Build history of the part. All positions in model axes, mm. A direction names the side the tool comes from. Coordinates: 2 decimals unless noted, no trailing zeros. Order: outer loops, then holes, each group sorted by start corner. A loop starts at its lowest first (then second) coordinate and runs counter-clockwise, first axis right, second up. Notation, with made-up numbers: (72, 53.25) - (78, 53.25) arc R12 ccw to (78, 67.25) - close; hole circle Ø1 at (19, -2.5). An arc over 180 degrees is marked (long way). Write each question's results on one line, items separated by ' | '.
from build123d import *

# Parameters (mm, degrees)
SKETCH_1_W           = 235
SKETCH_1_H           = 35
SKETCH_1_R           = 1.6
EXTRUDE_1_DEPTH      = 18
FILLET_1_R           = 1.5
CUT_EXTRUDE_1_DEPTH  = 237.337153237
SKETCH_3_W           = 13
SKETCH_3_H           = 19
CUT_EXTRUDE_2_DEPTH  = 237.337153237
SKETCH_5_R           = 1.6
CUT_EXTRUDE_5_DEPTH  = 121.151987083
SKETCH_6_R           = 3
CUT_EXTRUDE_6_DEPTH  = 10
SKETCH_10_W          = 29
SKETCH_10_H          = 35
CUT_EXTRUDE_9_DEPTH  = 30
FILLET_2_R           = 3
FILLET_5_R           = 1.5
SKETCH_11_W          = 30
SKETCH_11_H          = 19
CUT_EXTRUDE_10_DEPTH = 30
FILLET_6_R           = 5
EXTRUDE_2_DEPTH      = 10
SKETCH_13_W          = 250
SKETCH_13_H          = 88
CUT_EXTRUDE_11_DEPTH = 168.142155066


with BuildPart() as part:
    # 草图1 → 凸台-拉伸1 (new body)
    with BuildSketch(Plane.XY):
        Rectangle(SKETCH_1_W, SKETCH_1_H)
        with Locations((-47.5, 13.5)):
            Circle(SKETCH_1_R, mode=Mode.SUBTRACT)
        with Locations(Location((47.5, 13.5, 0), (0, 0, 180))):
            Circle(SKETCH_1_R, mode=Mode.SUBTRACT)
        with Locations((-47.5, 6)):
            Circle(SKETCH_1_R, mode=Mode.SUBTRACT)
        with Locations(Location((47.5, 6, 0), (0, 0, 180))):
            Circle(SKETCH_1_R, mode=Mode.SUBTRACT)
    extrude(amount=EXTRUDE_1_DEPTH)

    # 圆角1
    fillet_1_edges = [part.edges().sort_by_distance(p)[0] for p in [
        (-117.5, 17.5, 9),
        (117.5, 17.5, 9),
    ]]
    fillet(fillet_1_edges, radius=FILLET_1_R)

    # 草图2 → 切除-拉伸1 (cut, through all)
    with BuildSketch(Plane.ZY.offset(117.5)):
        Polygon((0, 1.5), (8, 17.5), (0, 17.5), align=None)
    extrude(amount=-CUT_EXTRUDE_1_DEPTH, mode=Mode.SUBTRACT)

    # 草图3 → 切除-拉伸2 (cut, through all)
    with BuildSketch(Plane.ZY.offset(117.5)):
        with Locations((11.5, -8)):
            Rectangle(SKETCH_3_W, SKETCH_3_H)
    extrude(amount=-CUT_EXTRUDE_2_DEPTH, mode=Mode.SUBTRACT)

    # 草图5 → 切除-拉伸5 (cut, through all)
    with BuildSketch(Plane(origin=(0, 0, 0), x_dir=(-1, 0, 0), z_dir=(0, 0, -1))):
        with Locations((47.5, -4.5)):
            Circle(SKETCH_5_R)
        with Locations((47.5, -12)):
            Circle(SKETCH_5_R)
        with Locations(Location((-47.5, -12, 0), (0, 0, 90))):
            Circle(SKETCH_5_R)
        with Locations(Location((-47.5, -4.5, 0), (0, 0, 90))):
            Circle(SKETCH_5_R)
    extrude(amount=-CUT_EXTRUDE_5_DEPTH, mode=Mode.SUBTRACT)

    # 草图6 → 切除-拉伸6 (cut)
    with BuildSketch(Plane(origin=(0, 0, 0), x_dir=(-1, 0, 0), z_dir=(0, 0, -1))):
        with Locations((47.5, 6)):
            Circle(SKETCH_6_R)
        with Locations((47.5, 13.5)):
            Circle(SKETCH_6_R)
        with Locations((-47.5, 6)):
            Circle(SKETCH_6_R)
        with Locations((-47.5, 13.5)):
            Circle(SKETCH_6_R)
    extrude(amount=-CUT_EXTRUDE_6_DEPTH, mode=Mode.SUBTRACT)

    # 草图10 → 切除-拉伸9 (cut)
    with BuildSketch(Plane(origin=(0, 0, 0), x_dir=(-1, 0, 0), z_dir=(0, 0, -1))):
        with Locations((-103, 0)):
            Rectangle(SKETCH_10_W, SKETCH_10_H)
    extrude(amount=-CUT_EXTRUDE_9_DEPTH, mode=Mode.SUBTRACT)

    # 圆角2
    fillet_2_edges = [part.edges().sort_by_distance(p)[0] for p in [
        (88.5, -17.5, 2.5),
        (-117.5, -17.5, 2.5),
    ]]
    fillet(fillet_2_edges, radius=FILLET_2_R)

    # 圆角5
    fillet_5_edges = [part.edges().sort_by_distance(p)[0] for p in [
        (88.5, 17.5, 13),
    ]]
    fillet(fillet_5_edges, radius=FILLET_5_R)

    # 草图11 → 切除-拉伸10 (cut)
    with BuildSketch(Plane(origin=(0, 0, 0), x_dir=(-1, 0, 0), z_dir=(0, 0, -1))):
        with Locations((0, -8)):
            Rectangle(SKETCH_11_W, SKETCH_11_H)
    extrude(amount=-CUT_EXTRUDE_10_DEPTH, mode=Mode.SUBTRACT)

    # 圆角6
    fillet_6_edges = [part.edges().sort_by_distance(p)[0] for p in [
        (15, 1.5, 2.5),
        (-15, -17.5, 2.5),
        (15, -17.5, 2.5),
        (-15, 1.5, 2.5),
    ]]
    fillet(fillet_6_edges, radius=FILLET_6_R)

    # 草图12 → 凸台-拉伸2 (add)
    with BuildSketch(Plane(origin=(60, 0, 0), x_dir=(0, 0, -1), z_dir=(1, 0, 0))):
        Polygon((-18, 1.5), (-5, -17.5), (-5, 1.5), align=None)
    extrude_2 = extrude(amount=EXTRUDE_2_DEPTH)

    # 镜向1: 凸台-拉伸2 across plane
    add(extrude_2.mirror(Plane(origin=(0, 0, 0), x_dir=(0, 0, 1), z_dir=(1, 0, 0))))


with BuildPart() as body_2:
    # 镜向2: mirrored copy
    add(part.part.mirror(Plane.ZX.offset(-50)))


with BuildPart() as part_1:
    add(part.part)

    # 草图13 → 切除-拉伸11 (cut, through all)
    with BuildSketch(Plane(origin=(0, 0, 0), x_dir=(-1, 0, 0), z_dir=(0, 0, -1))):
        with Locations((13.680717654, 5.907187604)):
            Rectangle(SKETCH_13_W, SKETCH_13_H)
    extrude(amount=-CUT_EXTRUDE_11_DEPTH, mode=Mode.SUBTRACT)


solid = body_2.part
1. Probe line 1 (Y direction, x = -47.5, z = 15.25); line 2 (X direction, y = -106, z = 12.25); line 3 (X direction, y = -106, z = 4.25). List the from-to ranges inside material, lowest first.
Solved:
line 1: y = -117.5 to -115.1, -111.9 to -107.6, -104.4 to -101.5 | line 2: x = -117.5 to -49.1, -45.9 to 45.9, 49.1 to 88.5 | line 3: x = -117.5 to -50.5, -44.5 to 44.5, 50.5 to 88.5
2. Band-saw the part on C-C on x = -5. Give the cut face in (y, z).
Solved:
outline: (-117.5, 8) - (-101.5, 0) - (-101.5, 18) - (-117.5, 18) - close
3. Two-plate mould, pull along Y, no slides. Class faces 1 (the face through (45.974, -113.019, 13.944)), 2 (the face through (-16, -110, 18)), 3 (the face through (-16.43, -84, 2.54)): +Y half, -Y half, draft (parallel to the pull), parting line (faces both ways), or undercut.
Solved:
face 1: undercut | face 2: draft | face 3: +Y half
4. Band-saw the part on A-A on x = -88.5. Give the cut face in (y, z).
Solved:
outline: (-117.5, 8) - (-101.5, 0) - (-82.5, 0) - (-82.5, 5) - (-101.5, 5) - (-101.5, 18) - (-117.5, 18) - close
5. Band-saw the part on B-B on x = -66.5. Give the cut face in (y, z), then the cut area to 4 significant figures.
Solved:
outline: (-117.5, 8) - (-101.5, 0) - (-82.5, 0) - (-82.5, 5) - (-101.5, 18) - (-117.5, 18) - close | area: 442.5 mm2
6. Drop flat-ended pins along their axis: pin 1 Ø5 at (x, y) = (47.5, -113.5) entering from -Z; pin 2 Ø3 at (x, y) = (-94, -104.5) entering from -Z; pin 3 Ø6.5 at (y, z) = (-94, 10) entering from -X. Give the stop position or say it passes through.
Solved:
pin 1: stops at z = 10 | pin 2: stops at z = 0.75 | pin 3: stops at x = -70
7. Tool access for faces 4 (the face through (-35, -92, 5)), 5 (the face through (-49, -105, 10)), 6 (the face through (79, -92, 5)), 7 (the face through (13.57, -100, 2.54)): list every direction of +Z, -Z, +X, -X, +Y, -Y with a clear straight run to the whole face (end or side of a thin tool).
Solved:
face 4: +Z, +Y | face 5: -Z | face 6: +Z, +X, +Y | face 7: +Z, -Z, +Y
